Work out the finished part from the listing and answer in its coordinate system (mm). A direction names the side the tool comes from. Coordinates: 2 decimals unless noted, no trailing zeros. Loops run counter-clockwise (first coordinate to the right, second up) from the corner with the lowest first, then second, coordinate; pieces in that order, holes last. Notation, with made-up numbers: (54.5, 10) -> (86.5, 10) arc R21 cw to (86.5, 42) -> close; hole circle Ø4 at (55, 30). An arc over 180 degrees is marked (long way). Use a Markdown table: item, result. Add a question column.
```python
from build123d import *

# Parameters (mm, degrees)
SKETCH_W     = 20.4
SKETCH_H     = 37.336792
PAD_DEPTH    = 7
POCKET_DEPTH = 7
CHAMFER_SIZE = 2


with BuildPart() as part:
    # Sketch → Pad (new body)
    with BuildSketch(Plane.XY):
        Rectangle(SKETCH_W, SKETCH_H)
        Polygon((3.85, 3.331604), (7.7, 10), (3.85, 16.668396), (-3.85, 16.668396), (-7.7, 10), (-3.85, 3.331604), align=None, mode=Mode.SUBTRACT)
    extrude(amount=PAD_DEPTH)

    # Sketch001 → Pocket (cut)
    with BuildSketch(Plane.XY.offset(7)):
        with BuildLine():
            Line((0, 14.5), (14, 14.5))
            Line((14, 14.5), (14, 5.5))
            Line((14, 5.5), (0, 5.5))
            ThreePointArc((0, 14.5), (-4.5, 10), (0, 5.5))
        make_face()
    pocket = extrude(amount=-POCKET_DEPTH, mode=Mode.SUBTRACT)

    # Mirrored: Pocket across Sketch001 H_Axis
    add(pocket.mirror(Plane(origin=(0, 0, 7), x_dir=(0, 0, 1), z_dir=(0, 1, 0))), mode=Mode.SUBTRACT)

    # Chamfer
    chamfer_edges = [part.edges().sort_by_distance(p)[0] for p in [
        (10.2, 18.668396, 3.5),
        (10.2, 14.5, 3.5),
        (10.2, 5.5, 3.5),
        (10.2, -5.5, 3.5),
        (10.2, -14.5, 3.5),
        (10.2, -18.668396, 3.5),
        (-10.2, -18.668396, 3.5),
        (-10.2, 18.668396, 3.5),
    ]]
    chamfer(chamfer_edges, length=CHAMFER_SIZE)


solid = part.part
```
Item 1: For faces 4 (the face through (-9.19, 17.68, 3.45)), 5 (the face through (9.2, -4.5, 3.5)), 6 (the face through (0, 16.668, 3)), determine the directions among +Z, -Z, +X, -X, +Y, -Y from which every point of the face is accessible in a straight line to the end or side of a thin tool.
Item 2: Section B-B (z = 3.75) is taken. Determine the outline of the cut face in (x, y).
Item 3: Find the intervals of material crossed by probe 1 along Y at (x, z) = (5.75, 2); probe 2 along Y at (x, z) = (2.25, 3.5); probe 3 along Y at (x, z) = (-5.25, 1.25), in increasing order.
Item 4: Section A-A (x = 7.75) is taken. Determine the outline of the cut face in (y, z).
Item 5: Section D-D (y = -10) is taken. Determine the outline of the cut face in (x, z).
Item 6: Section C-C (x = 3.25) is taken. Determine the outline of the cut face in (y, z).
Item 7: For a pull along Y with two mould halves and no side action, classify faces 1 (the face through (-9.19, -17.68, 3.45)), 2 (the face through (4, -14.5, 4)), 3 (the face through (-2, 0, 7)) as +Y half, -Y half, draft (parallel to the pull), parting line (faces both ways), or undercut.
Output:
| question | item | result |
|---|---|---|
| 1 | face 4 | +Z, -Z, -X, +Y |
| 1 | face 5 | +Z, -Z, +X |
| 1 | face 6 | +Z, -Z |
| 2 | outline | (-10.2, -16.67) -> (-8.2, -18.67) -> (8.2, -18.67) -> (10.2, -16.67) -> (10.2, -16.5) -> (8.2, -14.5) -> (0, -14.5) arc R4.5 cw to (0, -5.5) -> (8.2, -5.5) -> (10.2, -3.5) -> (10.2, 3.5) -> (8.2, 5.5) -> (5.1, 5.5) -> (3.85, 3.33) -> (-3.85, 3.33) -> (-7.7, 10) -> (-3.85, 16.67) -> (3.85, 16.67) -> (5.1, 14.5) -> (8.2, 14.5) -> (10.2, 16.5) -> (10.2, 16.67) -> (8.2, 18.67) -> (-8.2, 18.67) -> (-10.2, 16.67) -> close |
| 3 | probe 1 | y = -18.67 to -14.5, -5.5 to 5.5, 14.5 to 18.67 |
| 3 | probe 2 | y = -18.67 to -14.5, -5.5 to 3.33, 16.67 to 18.67 |
| 3 | probe 3 | y = -18.67 to 5.76, 14.24 to 18.67 |
| 4 | outline | (-18.67, 0) -> (-14.5, 0) -> (-14.5, 7) -> (-18.67, 7) -> close; (-5.5, 0) -> (5.5, 0) -> (5.5, 7) -> (-5.5, 7) -> close; (14.5, 0) -> (18.67, 0) -> (18.67, 7) -> (14.5, 7) -> close |
| 5 | outline | (-10.2, 0) -> (-4.5, 0) -> (-4.5, 7) -> (-10.2, 7) -> close |
| 6 | outline | (-18.67, 0) -> (-14.5, 0) -> (-14.5, 7) -> (-18.67, 7) -> close; (-5.5, 0) -> (3.33, 0) -> (3.33, 7) -> (-5.5, 7) -> close; (16.67, 0) -> (18.67, 0) -> (18.67, 7) -> (16.67, 7) -> close |
| 7 | face 1 | -Y half |
| 7 | face 2 | undercut |
| 7 | face 3 | draft |
